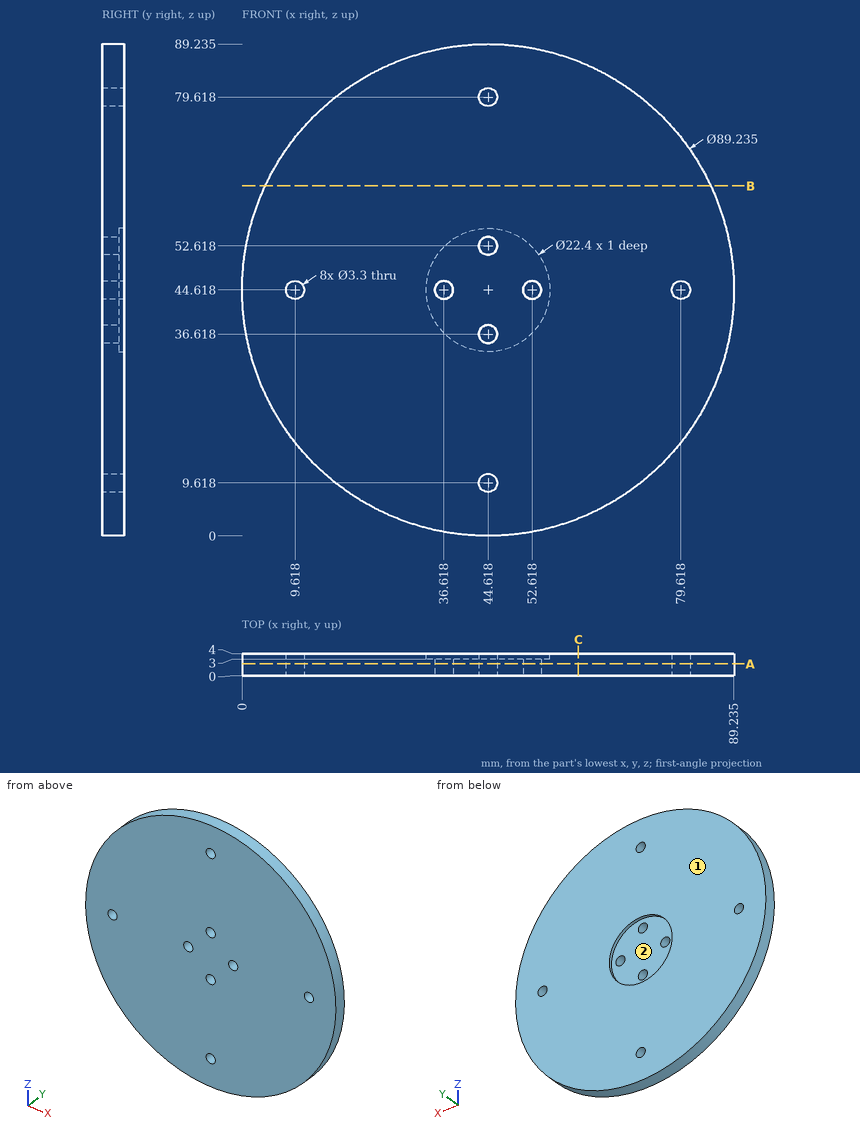
Design review of the part shown in the three views and the two pictorial views. Dimensions are in mm from the part's minimum x, y and z. Coordinates: 2 decimals unless noted, no trailing zeros. Write each loop counter-clockwise with the first axis right and the second up, starting at its lowest first coordinate (ties: lowest second). Pieces come first, ordered by that corner, then holes. Notation, with made-up numbers: (46, 55.5) -> (103, 55.5) arc R9 ccw to (103, 59.5) -> close; hole circle Ø1 at (76, 75). An arc over 180 degrees is marked (long way). Answer in a Markdown table with one row per item.
1. We need section B-B, the plane z = 63.5. State the section outline as (x, y) points.
Answers below:
| item | result |
|---|---|
| outline | (4.19, 0) -> (85.04, 0) -> (85.04, 4) -> (4.19, 4) -> close |
2. We need section A-A, the plane y = 2.2. Give the number of separate pieces and of enclosed holes in the cut face, and give its area (3 significant figures).
Answers below:
| item | result |
|---|---|
| separate pieces | 1 |
| enclosed holes | 8 |
| area | 6,190 mm^2 |
3. Draft analysis for pull direction X (two halves, no side actions). For the marked faces 1 and 2, state which applies: +X half, -X half, draft (parallel to the pull), parting line (faces both ways), or undercut.
Answers below:
| item | result |
|---|---|
| face 1 | draft |
| face 2 | undercut |
4. Clearance check with flat-ended pins moving along their axes: pin 1 Ø3 at (x, z) = (44.62, 79.62) entering from -Y; pin 2 Ø18 at (x, z) = (44.62, 44.62) entering from +Y; pin 3 Ø2 at (y, z) = (2, 74.5) entering from +X (1 decimal). State where each tip first meets the part, or that it passes through.
Answers below:
| item | result |
|---|---|
| pin 1 | passes through |
| pin 2 | stops at y = 3 |
| pin 3 | stops at x = 78.6 |
5. Wall thickness on probe 1 along Y at (x, z) = (46, 48.5); probe 2 along Z at (x, y) = (35.5, 0.65) (1 decimal); probe 3 along X at (y, z) = (3.45, 60.5): over which ranges is each line inside the solid? List them lowest first. Write a range as [from, to].
Answers below:
| item | result |
|---|---|
| probe 1 | y = [0, 3] |
| probe 2 | z = [0.9, 43.4], [45.8, 88.3] |
| probe 3 | x = [2.92, 86.31] |
6. We need section C-C, the plane x = 61. State the section outline as (y, z) points, and give its area (3 significant figures).
Answers below:
| item | result |
|---|---|
| outline | (0, 3.12) -> (4, 3.12) -> (4, 86.12) -> (0, 86.12) -> close |
| area | 332 mm^2 |
